Design review of the part built by this model. Coordinates are the model's own, in mm. Give positions to 0.01 mm unless a question says otherwise; leave off trailing zeros. Write each loop counter-clockwise with the first axis right and the second up, starting at its lowest first coordinate (ties: lowest second). Pieces come first, ordered by that corner, then holes. Notation, with made-up numbers: (37.25, 42.5) -> (53.25, 42.5) arc R23 ccw to (53.25, 80.5) -> close; hole circle Ø7 at (-8.5, 34). An arc over 180 degrees is marked (long way). Answer as a JSON object with one key per item and string values.
```python
from build123d import *

# Parameters (mm, degrees)
SKETCH1_W           = 40
SKETCH1_H           = 280
BOSS_EXTRUDE1_DEPTH = 4
SKETCH3_R           = 8
BOSS_EXTRUDE2_DEPTH = 4
SKETCH3_2_R         = 8
CUT_EXTRUDE1_DEPTH  = 4


with BuildPart() as part:
    # Sketch1 → Boss-Extrude1 (new body)
    with BuildSketch(Plane.XY):
        Rectangle(SKETCH1_W, SKETCH1_H)
    extrude(amount=BOSS_EXTRUDE1_DEPTH)

    # Sketch3 → Boss-Extrude2 (add)
    with BuildSketch(Plane(origin=(0, 0, 0), x_dir=(-1, 0, 0), z_dir=(0, 0, -1))):
        with Locations((0, 70)):
            Circle(SKETCH3_R)
        with Locations((0, -70)):
            Circle(SKETCH3_R)
    extrude(amount=-BOSS_EXTRUDE2_DEPTH)

    # Sketch3<2> → Cut-Extrude1 (cut)
    with BuildSketch(Plane(origin=(0, 0, 0), x_dir=(-1, 0, 0), z_dir=(0, 0, -1))):
        with Locations((0, 70)):
            Circle(SKETCH3_2_R)
        with Locations((0, -70)):
            Circle(SKETCH3_2_R)
    extrude(amount=-CUT_EXTRUDE1_DEPTH, mode=Mode.SUBTRACT)


solid = part.part
```
(1) For line 1 along Y through (x, z) = (0, 2); line 2 along X through (y, z) = (-70.5, 2.2); line 3 along Y through (x, z) = (-6.5, 2.8), list the stretches that pass through material, from the lowest coordinate up.
Here are the results:
{"line 1": "y = -140 to -78, -62 to 62, 78 to 140", "line 2": "x = -20 to -7.98, 7.98 to 20", "line 3": "y = -140 to -74.66, -65.34 to 65.34, 74.66 to 140"}
(2) We need section A-A, the plane x = 0. State the section outline as (y, z) points, then the cut area to 3 significant figures.
Here are the results:
{"outline": "(-140, 0) -> (-78, 0) -> (-78, 4) -> (-140, 4) -> close; (-62, 0) -> (62, 0) -> (62, 4) -> (-62, 4) -> close; (78, 0) -> (140, 0) -> (140, 4) -> (78, 4) -> close", "area": "992 mm²"}
(3) The part is to be moulded in two halves that separate along X. For faces 1 (the flat face through (0, 2, 4)), 2 (the cylindrical face through (1.041, -62.068, 1.972)), 3 (the cylindrical face through (1.041, 77.932, 1.972)), say which applies: +X half, -X half, draft (parallel to the pull), parting line (faces both ways), or undercut.
Here are the results:
{"face 1": "draft", "face 2": "undercut", "face 3": "undercut"}
(4) We need section B-B, the plane y = 70. State the section outline as (x, z) points.
Here are the results:
{"outline": "(-20, 0) -> (-8, 0) -> (-8, 4) -> (-20, 4) -> close; (8, 0) -> (20, 0) -> (20, 4) -> (8, 4) -> close"}
(5) We need section C-C, the plane z = 2.75. State the section outline as (x, y) points, then the cut area to 3 significant figures.
Here are the results:
{"outline": "(-20, -140) -> (20, -140) -> (20, 140) -> (-20, 140) -> close; hole circle Ø16 at (0, -70); hole circle Ø16 at (0, 70)", "area": "10,800 mm²"}
(6) Clearance check with a flat-ended pin moving along its axis: pin 1 (9.5 mm diameter, centred on x = 0, y = -70, fed in from +Z). State where the tip first meets the part, or that it passes through.
Here are the results:
{"pin 1": "passes through"}
